The figure shows three views and two pictorial views of one solid part (mm, origin at its lowest corner). Answer the questions. Round coordinates to 2 decimals unless told otherwise and drop trailing zeros. Order: outer loops, then holes, each group sorted by start corner. A loop starts at its lowest first (then second) coordinate and runs counter-clockwise, first axis right, second up. Notation, with made-up numbers: (-36.5, -25) -> (19.5, -25) arc R12 cw to (19.5, -3) -> close; hole circle Ø9 at (-4.75, -37). An arc over 180 degrees is marked (long way). Answer in a Markdown table with one row per item. Add a question column.
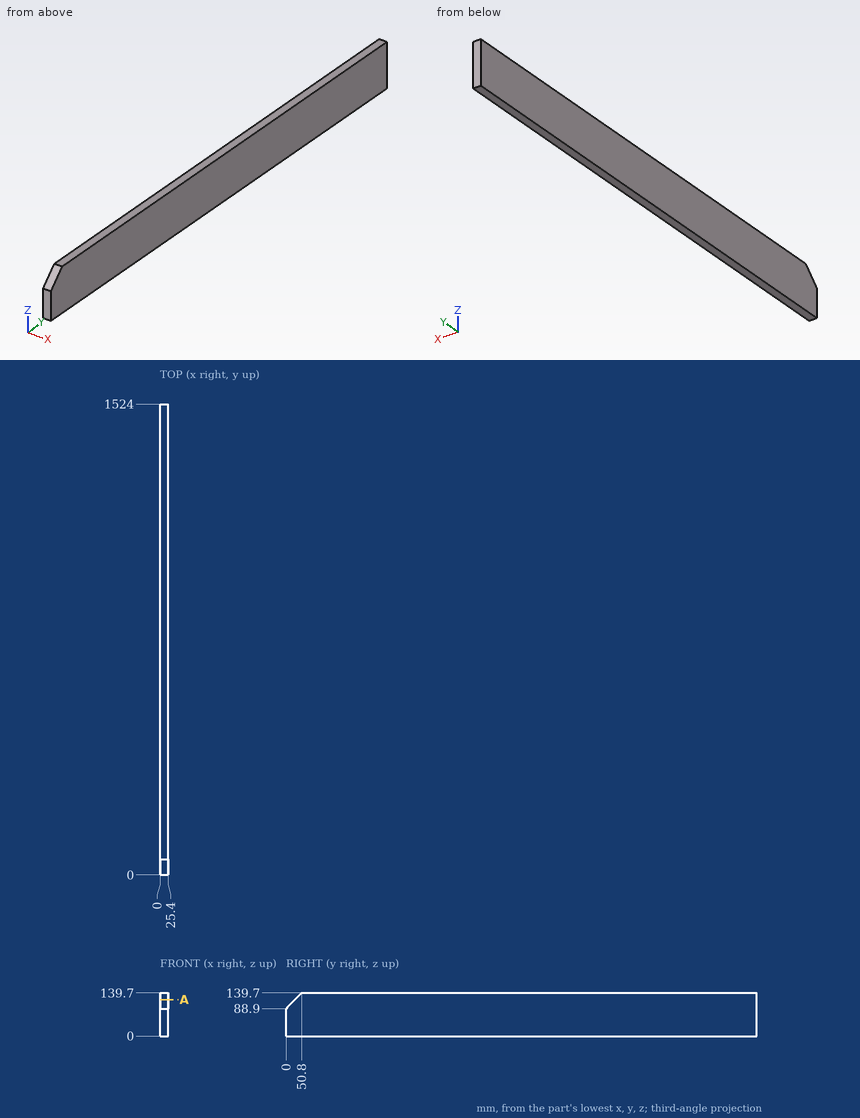
1. Straight lines are drawn through the part: line 1 along Y through (x, z) = (5.25, 114.5); line 2 along Y through (x, z) = (4.5, 111). For each, find the intervals that lie inside material, in ascending order.
2. This flat-tipped pin is pushed along its axis until it touches: pin 1 (1 mm diameter, centred on x = 14, z = 99, fed in from -Y). Where does it stop, or does it pass through?
3. The part is cut by section A-A (z = 118). Give the vertices of the cut face in (x, y), then the cut area to 3 significant figures.
Report:
| question | item | result |
|---|---|---|
| 1 | line 1 | y = 25.6 to 1524 |
| 1 | line 2 | y = 22.1 to 1524 |
| 2 | pin 1 | stops at y = 9.6 |
| 3 | outline | (0, 29.1) -> (25.4, 29.1) -> (25.4, 1524) -> (0, 1524) -> close |
| 3 | area | 38,000 mm^2 |
